Geometry: final body of the model. Coordinates: model frame, mm. Coordinates: 2 decimals unless noted, no trailing zeros. Answer as a JSON object with one key per item and string values. Group by question number.
Item 1: Section A-A on z = 2.3. State how many separate pieces and enclosed holes the cut face has, and give its area (3 significant figures).
Item 2: Line query: line 1 along Y through (x, z) = (-5, 1.4); line 2 along Y through (x, z) = (36, 2.05); line 3 along X through (y, z) = (-5.25, 0.35). Output: solid intervals per line, ascending. Write a range as from..to.
Item 3: Mould query, pull axis Z, two halves, no side actions, for faces 1 (the flat face through (2, 0, 3)), 2 (the cylindrical face through (-113, -9, 1)), 3 (the flat face through (2, 0, 0)). Classes: pulls with the +Z half, pulls with the -Z half, needs draft (parallel to the pull), parting line crosses it, or undercut.
```python
from build123d import *

# Parameters (mm, degrees)
SKETCH1_R           = 1.5
BOSS_EXTRUDE1_DEPTH = 3


with BuildPart() as part:
    # Sketch1 → Boss-Extrude1 (new body)
    with BuildSketch(Plane.XY):
        with BuildLine():
            Line((-110, 10), (110, 10))
            ThreePointArc((110, 10), (113.535533906, 8.535533906), (115, 5))
            Line((115, 5), (115, -5))
            ThreePointArc((115, -5), (113.535533906, -8.535533906), (110, -10))
            Line((110, -10), (-110, -10))
            ThreePointArc((-110, -10), (-113.535533906, -8.535533906), (-115, -5))
            Line((-115, -5), (-115, 5))
            ThreePointArc((-115, 5), (-113.535533906, 8.535533906), (-110, 10))
        make_face()
        with Locations((-105, 0)):
            Circle(SKETCH1_R, mode=Mode.SUBTRACT)
        with Locations((-95, 0)):
            Circle(SKETCH1_R, mode=Mode.SUBTRACT)
        with Locations((-85, 0)):
            Circle(SKETCH1_R, mode=Mode.SUBTRACT)
        with Locations((-75, 0)):
            Circle(SKETCH1_R, mode=Mode.SUBTRACT)
        with Locations((-65, 0)):
            Circle(SKETCH1_R, mode=Mode.SUBTRACT)
        with Locations((-55, 0)):
            Circle(SKETCH1_R, mode=Mode.SUBTRACT)
        with Locations((-45, 0)):
            Circle(SKETCH1_R, mode=Mode.SUBTRACT)
        with Locations((-35, 0)):
            Circle(SKETCH1_R, mode=Mode.SUBTRACT)
        with Locations((-25, 0)):
            Circle(SKETCH1_R, mode=Mode.SUBTRACT)
        with Locations((-15, 0)):
            Circle(SKETCH1_R, mode=Mode.SUBTRACT)
        with Locations((-5, 0)):
            Circle(SKETCH1_R, mode=Mode.SUBTRACT)
        with Locations((15, 0)):
            Circle(SKETCH1_R, mode=Mode.SUBTRACT)
        with Locations((25, 0)):
            Circle(SKETCH1_R, mode=Mode.SUBTRACT)
        with Locations((5, 0)):
            Circle(SKETCH1_R, mode=Mode.SUBTRACT)
        with Locations((35, 0)):
            Circle(SKETCH1_R, mode=Mode.SUBTRACT)
        with Locations((45, 0)):
            Circle(SKETCH1_R, mode=Mode.SUBTRACT)
        with Locations((55, 0)):
            Circle(SKETCH1_R, mode=Mode.SUBTRACT)
        with Locations((65, 0)):
            Circle(SKETCH1_R, mode=Mode.SUBTRACT)
        with Locations((75, 0)):
            Circle(SKETCH1_R, mode=Mode.SUBTRACT)
        with Locations((85, 0)):
            Circle(SKETCH1_R, mode=Mode.SUBTRACT)
        with Locations((95, 0)):
            Circle(SKETCH1_R, mode=Mode.SUBTRACT)
        with Locations((105, 0)):
            Circle(SKETCH1_R, mode=Mode.SUBTRACT)
    extrude(amount=BOSS_EXTRUDE1_DEPTH)


solid = part.part
```
Checks:
{
 "1": {"separate pieces": "1", "enclosed holes": "22", "area": "4,420 mm^2"},
 "2": {"line 1": "-10..-1.5, 1.5..10", "line 2": "-10..-1.12, 1.12..10", "line 3": "-114.99..114.99"},
 "3": {"face 1": "pulls with the +Z half", "face 2": "needs draft", "face 3": "pulls with the -Z half"}
}
